The listing builds one solid part. Answer for the finished solid, in the listing's coordinates (mm). Face numbers are marked on the shaded views. A direction names the side the tool comes from. Coordinates: 2 decimals unless noted, no trailing zeros. Write each loop counter-clockwise with the first axis right and the second up, starting at its lowest first coordinate (ties: lowest second). Pieces come first, ordered by that corner, then holes. Notation, with made-up numbers: M 74.25,-29.75 L 129.25,-29.75 A27 cw 129.25,-2.75 Z; hole C 0.25,35 d8. An arc over 180 degrees is marked long. Write item = value, one per line. Start each with the question number.
```python
from build123d import *

# Parameters (mm, degrees)
SKETCH_1_R          = 55
SKETCH_1_R_2        = 12
SKETCH_1_R_3        = 3
EXTRUDE_1_DEPTH     = 20
SKETCH_2_OUTSIDE_W  = 143.368
SKETCH_2_OUTSIDE_H  = 143.368
SKETCH_2_OUTSIDE_R  = 25
CUT_EXTRUDE_1_DEPTH = 10
SKETCH_4_R          = 5
CUT_EXTRUDE_2_DEPTH = 15
HOLE_WIZARD_M5_1_D  = 4.2


with BuildPart() as part:
    # 草图1 → 凸台-拉伸1 (new body)
    with BuildSketch(Plane.XY):
        Circle(SKETCH_1_R)
        Circle(SKETCH_1_R_2, mode=Mode.SUBTRACT)
        with Locations((47, 0)):
            Circle(SKETCH_1_R_3, mode=Mode.SUBTRACT)
        with Locations((23.5, -40.703193978)):
            Circle(SKETCH_1_R_3, mode=Mode.SUBTRACT)
        with Locations((-23.5, -40.703193978)):
            Circle(SKETCH_1_R_3, mode=Mode.SUBTRACT)
        with Locations((-47, 0)):
            Circle(SKETCH_1_R_3, mode=Mode.SUBTRACT)
        with Locations((-23.5, 40.703193978)):
            Circle(SKETCH_1_R_3, mode=Mode.SUBTRACT)
        with Locations((23.5, 40.703193978)):
            Circle(SKETCH_1_R_3, mode=Mode.SUBTRACT)
    extrude(amount=EXTRUDE_1_DEPTH)

    # 草图2 outside → 切除-拉伸1 (cut)
    with BuildSketch(Plane.XY):
        Rectangle(SKETCH_2_OUTSIDE_W, SKETCH_2_OUTSIDE_H)
        Circle(SKETCH_2_OUTSIDE_R, mode=Mode.SUBTRACT)
    extrude(amount=CUT_EXTRUDE_1_DEPTH, mode=Mode.SUBTRACT)

    # 草图4 → 切除-拉伸2 (cut)
    with BuildSketch(Plane.XY):
        with Locations((-47, 0)):
            Circle(SKETCH_4_R)
        with Locations((-23.5, 40.703193978)):
            Circle(SKETCH_4_R)
        with Locations((23.5, 40.703193978)):
            Circle(SKETCH_4_R)
        with Locations((47, 0)):
            Circle(SKETCH_4_R)
        with Locations((23.5, -40.703193978)):
            Circle(SKETCH_4_R)
        with Locations((-23.5, -40.703193978)):
            Circle(SKETCH_4_R)
    extrude(amount=CUT_EXTRUDE_2_DEPTH, mode=Mode.SUBTRACT)

    # M5 螺纹孔的螺纹孔钻头1 (through all)
    with Locations(Plane(origin=(0, 0, 0), x_dir=(-1, 0, 0), z_dir=(0, 0, -1))):
        with Locations((0, 18), (18, 0), (0, -18), (-18, 0)):
            Hole(HOLE_WIZARD_M5_1_D / 2)


solid = part.part
```
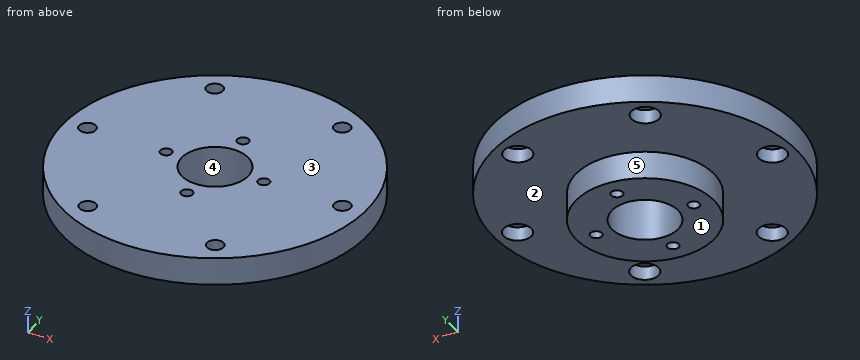
1. For the marked faces 1 and 2, determine the directions among +Z, -Z, +X, -X, +Y, -Y from which every point of the face is accessible in a straight line to the end or side of a thin tool.
2. Straight lines are drawn through the part: L1, parallel to X at y = -39.5, z = 15.5; L2, parallel to Y at x = 23.5, z = 17.45; L3, parallel to Y at x = 23.5, z = 11.4. For each, find the intervals that lie inside material, in ascending order. Write a range as [from, to].
3. The part is cut by section D-D, the plane y = 0. Count the separate pieces of the cut face and the enclosed holes in it, and give its area (3 significant figures).
4. The part is cut by section A-A, the plane x = 0. Write down the section's boundary in (y, z), and give its area (3 significant figures).
5. Each of these flat-tipped pins is pushed along its axis until it touches: pin 1 (11 mm diameter, centred on x = 25.5, y = -39, fed in from -Z); pin 2 (3 mm diameter, centred on x = 25.5, y = 41, fed in from -Z); pin 3 (4 mm diameter, centred on y = 5, z = 5.5, fed in from +X). Where does it stop, or does it pass through?
6. For a pull along X with two mould halves and no side action, classify the marked faces 3, 4 and 5 as pulls with the +X half, pulls with the -X half, needs draft (parallel to the pull), parting line crosses it, or undercut.
7. The part is cut by section B-B, the plane z = 8.25. Write down the section's boundary in (x, y), and give its area (3 significant figures).
8. The part is cut by section C-C, the plane x = -47. Write down the section's boundary in (y, z).
Solution:
q1.face_1 = -Z, +X, -X, +Y, -Y
q1.face_2 = -Z
q2.L1 = [-38.27, -26.25], [-20.75, 20.75], [26.25, 38.27]
q2.L2 = [-49.73, -43.7], [-37.7, 37.7], [43.7, 49.73]
q2.L3 = [-49.73, -45.7], [-35.7, 35.7], [45.7, 49.73]
q3.separate_pieces = 6
q3.enclosed_holes = 0
q3.area = 792 mm^2
q4.outline = M -55,10 L -25,10 L -25,0 L -20.1,0 L -20.1,20 L -55,20 Z; M -15.9,0 L -12,0 L -12,20 L -15.9,20 Z; M 12,0 L 15.9,0 L 15.9,20 L 12,20 Z; M 20.1,0 L 25,0 L 25,10 L 55,10 L 55,20 L 20.1,20 Z
q4.area = 952 mm^2
q5.pin_1 = 10
q5.pin_2 = 15
q5.pin_3 = 24.82
q6.face_3 = needs draft
q6.face_4 = undercut
q6.face_5 = parting line crosses it
q7.outline = C 0,0 d50; hole C -18,0 d4.2; hole C 0,0 d24; hole C 0,-18 d4.2; hole C 0,18 d4.2; hole C 18,0 d4.2
q7.area = 1,460 mm^2
q8.outline = M -28.57,10 L -5,10 L -5,15 L -3,15 L -3,20 L -28.57,20 Z; M 3,15 L 5,15 L 5,10 L 28.57,10 L 28.57,20 L 3,20 Z
